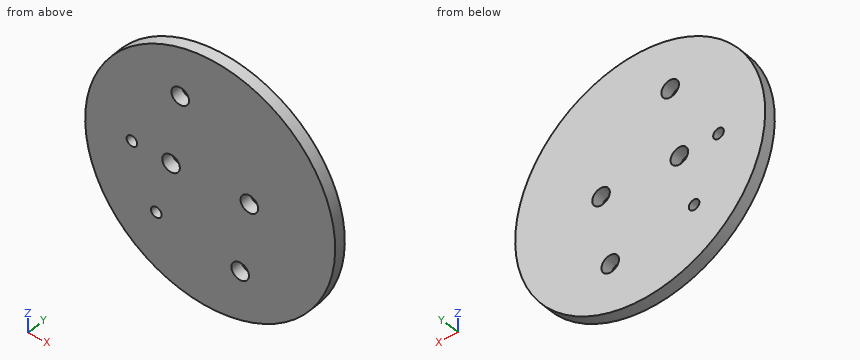
from build123d import *

# Parameters (mm, degrees)
SKETCH1_R                 = 50.673
SKETCH1_R_2               = 3.5687
BOSS_EXTRUDE1_DEPTH       = 4.7752
F_6_CLEARANCE_HOLE1_D     = 4.3053
F_6_CLEARANCE_HOLE1_DEPTH = 10.668
F_6_CLEARANCE_HOLE1_TIP   = 1.293442612


with BuildPart() as part:
    # Sketch1 → Boss-Extrude1 (new body)
    with BuildSketch(Plane(origin=(0, 0, 0), x_dir=(1, 0, 0), z_dir=(0, 1, 0))):
        with Locations(Location((0, 0, 0), (0, 0, 270))):
            Circle(SKETCH1_R)
        with Locations(Location((12.150198978, 29.333175157, 0), (0, 0, 270))):
            Circle(SKETCH1_R_2, mode=Mode.SUBTRACT)
        with Locations(Location((-12.150198978, -29.333175157, 0), (0, 0, 270))):
            Circle(SKETCH1_R_2, mode=Mode.SUBTRACT)
        with Locations(Location((-15.875, 0, 0), (0, 0, 270))):
            Circle(SKETCH1_R_2, mode=Mode.SUBTRACT)
        with Locations(Location((15.875, 0, 0), (0, 0, 270))):
            Circle(SKETCH1_R_2, mode=Mode.SUBTRACT)
    extrude(amount=BOSS_EXTRUDE1_DEPTH)

    # #6 Clearance Hole1
    with Locations(Plane(origin=(0, 4.7752, 0), x_dir=(1, 0, 0), z_dir=(0, 1, 0))):
        with Locations((-21.855257778, 23.03063628), (-31.739120068, -0.831118109)):
            Hole(F_6_CLEARANCE_HOLE1_D / 2, depth=F_6_CLEARANCE_HOLE1_DEPTH)
            with Locations((0, 0, -(F_6_CLEARANCE_HOLE1_DEPTH + F_6_CLEARANCE_HOLE1_TIP / 2))):  # 118° drill point
                Cone(0, F_6_CLEARANCE_HOLE1_D / 2, F_6_CLEARANCE_HOLE1_TIP, mode=Mode.SUBTRACT)


solid = part.part
CAD build for the part. Positions are in the model's coordinates, mm. Give positions to 0.01 mm unless a question says otherwise; leave off trailing zeros. Loops run counter-clockwise (first coordinate to the right, second up) from the corner with the lowest first, then second, coordinate; pieces in that order, holes last. Notation, with made-up numbers: M 59,-18 L 107,-18 A20 ccw 107,8 Z; hole C -29,-30.5 d2. An arc over 180 degrees is marked long. Answer in a Markdown table with one row per item. Add a question column.
Item 1: Band-saw the part on C-C on x = -31.5. Give the cut face in (y, z), then the cut area to 3 significant figures.
Item 2: Band-saw the part on B-B on y = 1.6. Give the cut face in (x, z) (3 decimals), then the cut area to 3 significant figures.
Item 3: Probe probe 1 along Z at (x, y) = (-14, 0.4); probe 2 along X at (y, z) = (3.75, 0); probe 3 along Z at (x, y) = (-23, 2.4). List the from-to ranges inside material, lowest first.
Item 4: Drop a flat-ended pin along its axis: P1, Ø1, axis at x = -1.5, y = 3, coming from the -Z side. Give the stop position or say it passes through.
Item 5: Band-saw the part on D-D on z = -15.5. Give the cut face in (x, y), then the cut area to 3 significant figures.
Item 6: Band-saw the part on A-A on z = 28. Give the cut face in (x, y), then the cut area to 3 significant figures.
Reply:
| question | item | result |
|---|---|---|
| 1 | outline | M 0,-39.69 L 4.78,-39.69 L 4.78,-1.31 L 0,-1.31 Z; M 0,2.97 L 4.78,2.97 L 4.78,39.69 L 0,39.69 Z |
| 1 | area | 359 mm^2 |
| 2 | outline | C 0,0 d101.346; hole C -31.739,0.831 d4.305; hole C -21.855,-23.031 d4.305; hole C -15.875,0 d7.137; hole C -12.15,29.333 d7.137; hole C 12.15,-29.333 d7.137; hole C 15.875,0 d7.137 |
| 2 | area | 7,880 mm^2 |
| 3 | probe 1 | z = -48.7 to -3.04, 3.04 to 26.28, 32.39 to 48.7 |
| 3 | probe 2 | x = -50.67 to -33.72, -29.75 to -19.44, -12.31 to 12.31, 19.44 to 50.67 |
| 3 | probe 3 | z = -45.15 to -24.85, -21.21 to 45.15 |
| 4 | P1 | stops at z = -50.66 |
| 5 | outline | M -48.24,0 L 48.24,0 L 48.24,4.78 L -48.24,4.78 Z |
| 5 | area | 461 mm^2 |
| 6 | outline | M -42.23,0 L -15.46,0 L -15.46,4.78 L -42.23,4.78 Z; M -8.84,0 L 42.23,0 L 42.23,4.78 L -8.84,4.78 Z |
| 6 | area | 372 mm^2 |
